Solid Edge part; units mm, degrees
sketch "Sketch1" plane through (0, 0, 0) normal (0, 0, 1) x (1, 0, 0)
  line L0 (0, 0) -> (-247.23, 0)
  line L1 (-247.23, 0) -> (-247.23, -85.2)
  line L2 (-247.23, -85.2) -> (0, -85.2)
  line L3 (0, -85.2) -> (0, 0)
extrude "Protrusion1" add sketch "Sketch1" against normal blind 20.1
sketch "Sketch2" plane through (-123.615, -42.6, 0) normal (0, 0, 1) x (1, 0, 0)
  circle A0 centre (154.995, -6.1) radius 55
extrude "ExtrudedCutout_1" cut sketch "Sketch2" against normal blind 21
fillet "Round_1" radius 3 1 edges at (0, 0, -10.05)
chamfer "Chamfer_1" distance 2 angle 45 1 edges at (-9.763, -85.2, -10.05)
sketch "Sketch3" plane through (-123.615, -42.6, 0) normal (0, 0, 1) x (1, 0, 0)
  circle A0 centre (57.505, -8.9) radius 6.6
extrude "ExtrudedCutout_2" cut sketch "Sketch3" against normal blind 22
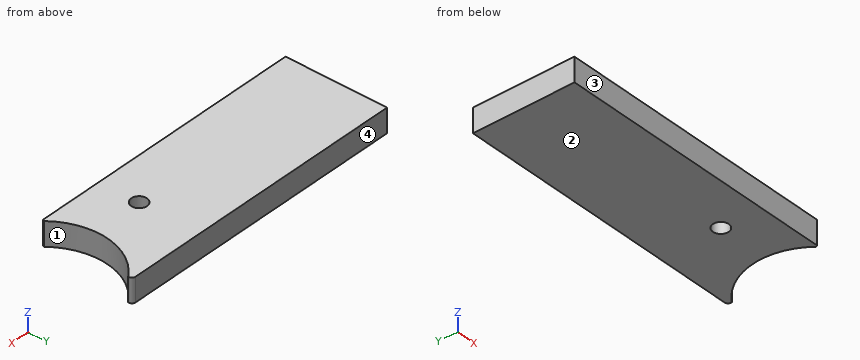
Source: CAD feature listing. Evaluate the final solid. Frame: model axes, mm. Face numbers are marked on the shaded views. Coordinates: 2 decimals unless noted, no trailing zeros. Loops run counter-clockwise (first coordinate to the right, second up) from the corner with the lowest first, then second, coordinate; pieces in that order, holes last. Notation, with made-up numbers: M 14.5,13.25 L 40.5,13.25 A30 ccw 40.5,52.25 Z; hole C 30,-23.5 d8. An arc over 180 degrees is marked long. Put each result on its own line as item: value. Start each with the question number.
1) Ray query, L1, parallel to Y at x = -66, z = -15.5; L2, parallel to X at y = -14.5, z = -1.75; L3, parallel to X at y = -54, z = -10. Return the intervals inside material, ascending. Write a range as from..to.
2) Cut plane D-D on y = -27.5. Return the cut outline in (x, z), then the cut area to 3 significant figures.
3) Cut plane C-C on z = -12.25. Return the cut outline in (x, y).
4) Pull-direction query (Y, two-part tool) for the marked faces 1, 2, 3 and 4; classes: pulls with the +Y half, pulls with the -Y half, needs draft (parallel to the pull), parting line crosses it, or undercut.
5) Cut plane B-B on y = -51.5. Return the cut outline in (x, z), then the cut area to 3 significant figures.
6) Cut plane A-A on x = -66.11. Return the cut outline in (y, z), then the cut area to 3 significant figures.
7) Contact query for flat-ended pins moving along their axis: pin 1 Ø17 at (x, y) = (-66.11, -51.5) entering from -Z; pin 2 Ø1 at (y, z) = (-46.5, -16.5) entering from +X; pin 3 Ø8 at (y, z) = (-40.5, -7.5) entering from +X; pin 4 Ø1.5 at (y, z) = (-76.5, -11.5) entering from +X. Output: stop coordinate, or through.
The answers:
1. L1: y = -85.2..-58.1, -44.9..0
1. L2: x = -247.23..-11.69
1. L3: x = -247.23..-72.22, -60..-23.36
2. outline: M -247.23,-20.1 L -19.37,-20.1 L -19.37,0 L -247.23,0 Z
2. area: 4,580 mm²
3. outline: M -247.23,-85.2 L -11.72,-85.2 L -11.02,-83.73 A55 cw 0,-3.53 L 0,-3 A3 ccw -3,0 L -247.23,0 Z; hole C -66.11,-51.5 d13.2
4. face 1: undercut
4. face 2: needs draft
4. face 3: pulls with the -Y half
4. face 4: pulls with the +Y half
5. outline: M -247.23,-20.1 L -72.71,-20.1 L -72.71,0 L -247.23,0 Z; M -59.51,-20.1 L -23.55,-20.1 L -23.55,0 L -59.51,0 Z
5. area: 4,230 mm²
6. outline: M -85.2,-20.1 L -58.1,-20.1 L -58.1,0 L -85.2,0 Z; M -44.9,-20.1 L 0,-20.1 L 0,0 L -44.9,0 Z
6. area: 1,450 mm²
7. pin 1: stops at z = -20.1
7. pin 2: stops at x = -23.55
7. pin 3: stops at x = -22.25
7. pin 4: stops at x = -15.63
